Part model, mm, in its own coordinate system. A direction names the side the tool comes from. Give positions to 0.01 mm unless a question says otherwise; leave off trailing zeros. Order: outer loops, then holes, each group sorted by start corner. A loop starts at its lowest first (then second) coordinate and runs counter-clockwise, first axis right, second up. Notation, with made-up numbers: (-33, 75) - (12, 75) arc R22 cw to (12, 81) - close; hole circle Ø3 at (1.5, 45.5). An arc over 180 degrees is marked (long way). One line per item, written item: value.
```python
from build123d import *

# Parameters (mm, degrees)
SKETCH006_R     = 3.15
PAD002_DEPTH    = 190
SKETCH011_R     = 5
PAD007_DEPTH    = 50
SKETCH010_R     = 5
PAD006_DEPTH    = 50
SKETCH008_R     = 13
PAD004_DEPTH    = 15
SKETCH009_R     = 9
PAD005_DEPTH    = 15
SKETCH013_R     = 6
PAD008_DEPTH    = 26
BOX001_W        = 50
BOX001_H        = 180
BOX001_DEPTH    = 20
SKETCH015_R     = 1.5
POCKET001_DEPTH = 395.766885
SKETCH016_R     = 1.5
POCKET002_DEPTH = 395.766885
SKETCH017_R     = 3
POCKET003_DEPTH = 5
SKETCH018_R     = 3
POCKET004_DEPTH = 5
SKETCH022_W     = 5
SKETCH022_H     = 20
POCKET008_DEPTH = 395.766885
SKETCH023_W     = 5
SKETCH023_H     = 20
POCKET009_DEPTH = 395.766885


with BuildPart() as pad002:
    # Sketch006 → Pad002 (new body)
    with BuildSketch(Plane.XZ.offset(80)):
        Circle(SKETCH006_R)
    extrude(amount=-PAD002_DEPTH)


with BuildPart() as pad007:
    # Sketch011 → Pad007 (new body)
    with BuildSketch(Plane.XZ.offset(-75)):
        Circle(SKETCH011_R)
    extrude(amount=PAD007_DEPTH)


with BuildPart() as scassi_perno:
    # Sketch010 → Pad006 (new body)
    with BuildSketch(Plane.XZ.offset(25)):
        Circle(SKETCH010_R)
    extrude(amount=PAD006_DEPTH)

    # Fusion002: union Pad007
    add(pad007.part)


with BuildPart() as scasso_ruota_dentata:
    # Sketch008 → Pad004 (new body)
    with BuildSketch(Plane.XZ.offset(-3)):
        Circle(SKETCH008_R)
    extrude(amount=PAD004_DEPTH)


with BuildPart() as obj1:
    # Sketch009 → Pad005 (new body)
    with BuildSketch(Plane.XZ.offset(-3)):
        with Locations((15.997087, 9e-06)):
            Circle(SKETCH009_R)
    extrude(amount=PAD005_DEPTH)

    # Fusion001: union scasso_ruota_dentata
    add(scasso_ruota_dentata.part)


with BuildPart() as fusion:
    # Sketch013 → Pad008 (new body)
    with BuildSketch(Plane.XZ.offset(11)):
        with Locations((16.059561, 9e-06)):
            Circle(SKETCH013_R)
    extrude(amount=PAD008_DEPTH)

    # Fusion005: union scassi_perno, obj1
    add(scassi_perno.part)
    add(obj1.part)

    # Fusion: union Pad002
    add(pad002.part)


with BuildPart() as mirrored007:
    # Box001 → Box001 (new body)
    with BuildSketch(Plane(origin=(-20, -88, -21), x_dir=(1, 0, 0), z_dir=(0, 0, 1))):
        with Locations((25, 90)):
            Rectangle(BOX001_W, BOX001_H)
    extrude(amount=BOX001_DEPTH)

    # Cut001: cut Fusion
    add(fusion.part, mode=Mode.SUBTRACT)

    # Sketch015 → Pocket001 (cut, through all)
    with BuildSketch(Plane(origin=(0, 0, -21), x_dir=(1, 0, 0), z_dir=(0, 0, -1))):
        with Locations((23, 70)):
            Circle(SKETCH015_R)
    pocket001 = extrude(amount=-POCKET001_DEPTH, mode=Mode.SUBTRACT)

    # Mirrored: Pocket001 across Sketch015 H_Axis
    add(pocket001.mirror(Plane(origin=(0, 0, -21), x_dir=(0, 0, -1), z_dir=(0, -1, 0))), mode=Mode.SUBTRACT)

    # Sketch016 → Pocket002 (cut, through all)
    with BuildSketch(Plane(origin=(0, 0, -21), x_dir=(1, 0, 0), z_dir=(0, 0, -1))):
        with Locations((-12, 70)):
            Circle(SKETCH016_R)
    pocket002 = extrude(amount=-POCKET002_DEPTH, mode=Mode.SUBTRACT)

    # Mirrored001: Pocket002 across Sketch016 H_Axis
    add(pocket002.mirror(Plane(origin=(0, 0, -21), x_dir=(0, 0, -1), z_dir=(0, -1, 0))), mode=Mode.SUBTRACT)

    # Sketch017 → Pocket003 (cut)
    with BuildSketch(Plane(origin=(0, 0, -21), x_dir=(1, 0, 0), z_dir=(0, 0, -1))):
        with Locations((23, 70)):
            Circle(SKETCH017_R)
    pocket003 = extrude(amount=-POCKET003_DEPTH, mode=Mode.SUBTRACT)

    # Mirrored002: Pocket003 across Sketch017 H_Axis
    add(pocket003.mirror(Plane(origin=(0, 0, -21), x_dir=(0, 0, -1), z_dir=(0, -1, 0))), mode=Mode.SUBTRACT)

    # Sketch018 → Pocket004 (cut)
    with BuildSketch(Plane(origin=(0, 0, -21), x_dir=(1, 0, 0), z_dir=(0, 0, -1))):
        with Locations((-12, 70)):
            Circle(SKETCH018_R)
    pocket004 = extrude(amount=-POCKET004_DEPTH, mode=Mode.SUBTRACT)

    # Mirrored003: Pocket004 across Sketch018 H_Axis
    add(pocket004.mirror(Plane(origin=(0, 0, -21), x_dir=(0, 0, -1), z_dir=(0, -1, 0))), mode=Mode.SUBTRACT)

    # Sketch022 → Pocket008 (cut, through all)
    with BuildSketch(Plane(origin=(0, 0, -21), x_dir=(1, 0, 0), z_dir=(0, 0, -1))):
        with Locations((22.5, 53)):
            Rectangle(SKETCH022_W, SKETCH022_H)
    pocket008 = extrude(amount=-POCKET008_DEPTH, mode=Mode.SUBTRACT)

    # Mirrored006: Pocket008 across Sketch022 H_Axis
    add(pocket008.mirror(Plane(origin=(0, 0, -21), x_dir=(0, 0, -1), z_dir=(0, -1, 0))), mode=Mode.SUBTRACT)

    # Sketch023 → Pocket009 (cut, through all)
    with BuildSketch(Plane(origin=(0, 0, -21), x_dir=(1, 0, 0), z_dir=(0, 0, -1))):
        with Locations((-11.5, 53)):
            Rectangle(SKETCH023_W, SKETCH023_H)
    pocket009 = extrude(amount=-POCKET009_DEPTH, mode=Mode.SUBTRACT)

    # Mirrored007: Pocket009 across Sketch023 H_Axis
    add(pocket009.mirror(Plane(origin=(0, 0, -21), x_dir=(0, 0, -1), z_dir=(0, -1, 0))), mode=Mode.SUBTRACT)


solid = mirrored007.part
```
1) Which spindle directions (+Z, -Z, +X, -X, +Y, -Y) get a long thin tool onto all of the face, cutting with end or side? Do faces 1 (the flat face through (-14, -53, -11)), 2 (the cylindrical face through (-0.06, 83.38, -3.15)), 3 (the flat face through (5, -88, -11)), 4 (the cylindrical face through (22.35, 67.07, -18.54)), 5 (the flat face through (16, -37, -3)). Say none if no direction does.
Outcome:
face 1: +Z, -Z
face 2: +Z, +Y
face 3: +Z, -Z, +X, -X, -Y
face 4: -Z
face 5: +Z
2) Mould opens along X. For faces 6 (the flat face through (-20, 1, -11)), 7 (the flat face through (22, -43, -11)), 8 (the flat face through (5, 92, -11)), 9 (the cylindrical face through (22.805, -71.487, -8.605)) say: released by +X, released by -X, zero draft, split by the parting line, or undercut.
Outcome:
face 6: released by -X
face 7: undercut
face 8: zero draft
face 9: undercut
3) Drill centre lines: line 1 along X through (y, z) = (-47, -15.5); line 2 along X through (y, z) = (70, -19.75); line 3 along Y through (x, z) = (-12, -18.5). Where is each one in solid material? Low to high. Write a range as from..to.
Outcome:
line 1: x = -20..-14, -9..20, 25..30
line 2: x = -20..-15, -9..20, 26..30
line 3: y = -88..-73, -67..-63, -43..43, 63..67, 73..92
4) Cut at B-B, the plane x = 18. Give the cut face in (y, z), then the cut area to 3 significant figures.
Outcome:
outline: (-88, -21) - (92, -21) - (92, -1) - (3, -1) - (3, -8.77) - (-12, -8.77) - (-12, -5.68) - (-37, -5.68) - (-37, -1) - (-88, -1) - close
area: 3,370 mm^2
5) Cut at A-A, the plane z = -18. Give the number of separate pieces and of enclosed holes in the cut face, then the cut area to 3 significant figures.
Outcome:
separate pieces: 1
enclosed holes: 8
area: 8,490 mm^2
6) Pin check, flat tips, straight feed: pin 1 (4 mm diameter, centred on x = -12, y = 70, fed in from -Z); pin 2 (1.5 mm diameter, centred on x = 16.5, y = -12.5, fed in from +Z). Stop position of each tip, or through.
Outcome:
pin 1: stops at z = -16
pin 2: stops at z = -5.88
